Part model, mm, in its own coordinate system. A direction names the side the tool comes from. Round coordinates to 2 decimals unless told otherwise and drop trailing zeros. Write each loop counter-clockwise with the first axis right and the second up, starting at its lowest first coordinate (ties: lowest second). Pieces come first, ordered by that corner, then holes.
```python
from build123d import *

# Parameters (mm, degrees)
SKETCH1_W               = 45
SKETCH1_H               = 30
SKETCH1_R               = 4
BOSS_EXTRUDE1_DEPTH     = 10
SKETCH2_R               = 2.5
BOSS_EXTRUDE2_DEPTH     = 2.5
MIRROR3_COPY_1_SKETCH_R = 2.5
MIRROR3_COPY_1_DEPTH    = 2.5


with BuildPart() as part:
    # Sketch1 → Boss-Extrude1 (new body)
    with BuildSketch(Plane(origin=(0, 0, 0), x_dir=(1, 0, 0), z_dir=(0, 1, 0))):
        Rectangle(SKETCH1_W, SKETCH1_H)
        with Locations(Location((0, 0, 0), (0, 0, 270))):
            Circle(SKETCH1_R, mode=Mode.SUBTRACT)
    extrude(amount=BOSS_EXTRUDE1_DEPTH)

    # Sketch2 → Boss-Extrude2 (add)
    with BuildSketch(Plane(origin=(22.5, 0, 0), x_dir=(0, 0, -1), z_dir=(1, 0, 0))):
        with BuildLine():
            Line((-15, 10), (15, 10))
            Line((15, 10), (15, 25))
            ThreePointArc((15, 25), (0, 40), (-15, 25))
            Line((-15, 25), (-15, 10))
        make_face()
        with Locations((0, 25)):
            Circle(SKETCH2_R, mode=Mode.SUBTRACT)
    boss_extrude2 = extrude(amount=-BOSS_EXTRUDE2_DEPTH)

    # Mirror2: Boss-Extrude2 across plane
    add(boss_extrude2.mirror(Plane(origin=(18.75, 0, 0), x_dir=(0, 0, 1), z_dir=(1, 0, 0))))

    # Mirror3: Boss-Extrude2 across plane
    add(boss_extrude2.mirror(Plane(origin=(0, 0, 0), x_dir=(0, 0, 1), z_dir=(1, 0, 0))))

    # Mirror3 copy 1 sketch → Mirror3 copy 1 (add)
    with BuildSketch(Plane(origin=(-15, 0, 0), x_dir=(0, 0, -1), z_dir=(1, 0, 0))):
        with BuildLine():
            Line((-15, 10), (15, 10))
            Line((15, 10), (15, 25))
            ThreePointArc((15, 25), (0, 40), (-15, 25))
            Line((-15, 25), (-15, 10))
        make_face()
        with Locations((0, 25)):
            Circle(MIRROR3_COPY_1_SKETCH_R, mode=Mode.SUBTRACT)
    extrude(amount=-MIRROR3_COPY_1_DEPTH)


solid = part.part
```
Q1. Drop flat-ended pins along their axis: pin 1 (7 mm diameter, centred on x = 0, z = 0, fed in from +Y); pin 2 (1.2 mm diameter, centred on x = 19, z = -2.5, fed in from +Y); pin 3 (10 mm diameter, centred on x = 11.5, y = 30, fed in from +Z). Give the stop position or say it passes through.
Values follow:
pin 1: passes through
pin 2: stops at y = 10
pin 3: stops at z = 14.93
Q2. Cut at D-D on z = -7.5. Write the cut outline in (x, y), plus the area to 3 significant figures.
Values follow:
outline: (-22.5, 0) - (22.5, 0) - (22.5, 37.99) - (20, 37.99) - (20, 10) - (17.5, 10) - (17.5, 37.99) - (15, 37.99) - (15, 10) - (-15, 10) - (-15, 37.99) - (-17.5, 37.99) - (-17.5, 10) - (-20, 10) - (-20, 37.99) - (-22.5, 37.99) - close
area: 730 mm2
Q3. Cut at A-A on x = 0. Write the cut outline in (y, z), plus the area to 3 significant figures.
Values follow:
outline: (0, -15) - (10, -15) - (10, -4) - (0, -4) - close; (0, 4) - (10, 4) - (10, 15) - (0, 15) - close
area: 220 mm2
Q4. Wall check: L1, parallel to X at y = 11, z = -10.5; L2, parallel to Y at x = -20.9, z = 0; L3, parallel to X at y = 2.75, z = 0. Give the ranges that are in metal, low to high.
Values follow:
L1: x = -22.5 to -20, -17.5 to -15, 15 to 17.5, 20 to 22.5
L2: y = 0 to 22.5, 27.5 to 40
L3: x = -22.5 to -4, 4 to 22.5
Q5. Cut at C-C on z = 0. State how many separate pieces and enclosed holes the cut face has, plus the area to 3 significant figures.
Values follow:
separate pieces: 6
enclosed holes: 0
area: 620 mm2
Q6. Cut at B-B on y = 30. Write the cut outline in (x, z), plus the area to 3 significant figures.
Values follow:
outline: (-22.5, -14.14) - (-20, -14.14) - (-20, 14.14) - (-22.5, 14.14) - close; (-17.5, -14.14) - (-15, -14.14) - (-15, 14.14) - (-17.5, 14.14) - close; (15, -14.14) - (17.5, -14.14) - (17.5, 14.14) - (15, 14.14) - close; (20, -14.14) - (22.5, -14.14) - (22.5, 14.14) - (20, 14.14) - close
area: 283 mm2
Q7. Mould opens along X. For faces 3 (the flat face through (22.5, 20, 0)), 4 (the flat face through (-22.5, 20, 0)), 5 (the cylindrical face through (16.23, 27.48, 0.33)), 6 (the cylindrical face through (-3.905, 4.93, -0.867)) say: +X half, -X half, draft (parallel to the pull), parting line (faces both ways), or undercut.
Values follow:
face 3: +X half
face 4: -X half
face 5: draft
face 6: undercut
Q8. Which spindle directions (+Z, -Z, +X, -X, +Y, -Y) get a long thin tool onto all of the face, cutting with end or side? Do faces 1 (the flat face through (-20, 22, 0)), 2 (the cylindrical face through (16, 40, 0)). Say none if no direction does.
Values follow:
face 1: +Z, -Z, +Y
face 2: +X, -X, +Y
